Can you work these out from the model? Positions are in its coordinate system, mm. A direction names the side the tool comes from. Give positions to 0.01 mm unless a question says otherwise; leave off trailing zeros. Write each loop counter-clockwise with the first axis right and the second up, starting at its lowest first coordinate (ties: lowest second). Pieces come first, ordered by that corner, then holes. Notation, with made-up numbers: (42, 6.5) -> (89, 6.5) arc R14 cw to (89, 30.5) -> close; hole circle Ø10 at (9.5, 51). An arc over 180 degrees is marked (long way). Answer as CSV lines item,"result". Start each with the question number.
1. I'm going to push a flat-ended pin straight in: P1, Ø2.5, axis at x = -85, y = -64.5, coming from the +Z side. Where does the tip first touch, or does it pass through?
2. If we section it at A-A on x = -40: Write out the boundary of the cut face in (y, z).
3. I need wall thicknesses on line 1 (X direction, y = -32, z = 3.15); line 2 (X direction, y = 64.5, z = 2.4); line 3 (Y direction, x = -85, z = 2.05). Which ranges of each line are inside material? Lowest first, please. Write a range as [from, to].
4. On a 3-axis mill with a long thin cutter (end or side, diameter ignored), from which of +Z, -Z, +X, -X, +Y, -Y can I reach the whole of each face in a straight line? I mean faces 1 (the face through (-50.6, -28, 3)), 2 (the face through (-125, -1, 2)). Say none if no direction works.
5. If we section it at B-B on z = 2.2: Write out the boundary of the cut face in (x, y).
6. If we mould it in two halves opening along X, with no side actions, what happens to faces 3 (the face through (29.4, -27, 3)), 4 (the face through (50.6, -28, 3)), 5 (the face through (-2, 74.5, 2)), 6 (the face through (125, -1, 2))? For each: pulls with the +X half, pulls with the -X half, needs draft (parallel to the pull), parting line crosses it, or undercut.
```python
from build123d import *

# Parameters (mm, degrees)
ESQUISSE1_W             = 250
ESQUISSE1_H             = 149
BOSS_EXTRU_1_DEPTH      = 5
ESQUISSE2_R             = 1.5
ENL_V_MAT_EXTRU_1_DEPTH = 5
ENL_V_MAT_EXTRU_2_DEPTH = 5


with BuildPart() as part:
    # Esquisse1 → Boss.-Extru.1 (new body)
    with BuildSketch(Plane.XY):
        Rectangle(ESQUISSE1_W, ESQUISSE1_H)
    extrude(amount=BOSS_EXTRU_1_DEPTH)

    # Esquisse2 → Enlèv. mat.-Extru.1 (cut)
    with BuildSketch(Plane.XY.offset(5)):
        with Locations((-85, 64.5)):
            Circle(ESQUISSE2_R)
        with Locations(Location((-85, -64.5, 0), (0, 0, 180))):
            Circle(ESQUISSE2_R)
        with Locations((85, -64.5)):
            Circle(ESQUISSE2_R)
        with Locations(Location((85, 64.5, 0), (0, 0, 180))):
            Circle(ESQUISSE2_R)
    extrude(amount=-ENL_V_MAT_EXTRU_1_DEPTH, mode=Mode.SUBTRACT)

    # Esquisse3 → Enlèv. mat.-Extru.2 (cut)
    with BuildSketch(Plane.XY.offset(5)):
        with BuildLine():
            Line((-29.4, -12.5), (-29.4, -42.5))
            ThreePointArc((-29.4, -42.5), (-40, -53.1), (-50.6, -42.5))
            Line((-50.6, -42.5), (-50.6, -12.5))
            ThreePointArc((-50.6, -12.5), (-40, -1.9), (-29.4, -12.5))
        make_face()
        with BuildLine():
            Line((29.4, -12.5), (29.4, -42.5))
            ThreePointArc((29.4, -42.5), (40, -53.1), (50.6, -42.5))
            Line((50.6, -42.5), (50.6, -12.5))
            ThreePointArc((50.6, -12.5), (40, -1.9), (29.4, -12.5))
        make_face()
    extrude(amount=-ENL_V_MAT_EXTRU_2_DEPTH, mode=Mode.SUBTRACT)


solid = part.part
```
Computed values:
1,P1,"passes through"
2,outline,"(-74.5, 0) -> (-53.1, 0) -> (-53.1, 5) -> (-74.5, 5) -> close; (-1.9, 0) -> (74.5, 0) -> (74.5, 5) -> (-1.9, 5) -> close"
3,line 1,"x = [-125, -50.6], [-29.4, 29.4], [50.6, 125]"
3,line 2,"x = [-125, -86.5], [-83.5, 83.5], [86.5, 125]"
3,line 3,"y = [-74.5, -66], [-63, 63], [66, 74.5]"
4,face 1,"+Z, -Z"
4,face 2,"+Z, -Z, -X, +Y, -Y"
5,outline,"(-125, -74.5) -> (125, -74.5) -> (125, 74.5) -> (-125, 74.5) -> close; hole circle Ø3 at (-85, -64.5); hole circle Ø3 at (-85, 64.5); hole (-50.6, -42.5) arc R10.6 ccw to (-29.4, -42.5) -> (-29.4, -12.5) arc R10.6 ccw to (-50.6, -12.5) -> close; hole (29.4, -42.5) arc R10.6 ccw to (50.6, -42.5) -> (50.6, -12.5) arc R10.6 ccw to (29.4, -12.5) -> close; hole circle Ø3 at (85, -64.5); hole circle Ø3 at (85, 64.5)"
6,face 3,"undercut"
6,face 4,"undercut"
6,face 5,"needs draft"
6,face 6,"pulls with the +X half"
